Can you work these out from the model? Positions are in its coordinate system, mm. A direction names the side the tool comes from. Give positions to 0.01 mm unless a question says otherwise; leave off trailing zeros. Loops run counter-clockwise (first coordinate to the right, second up) from the corner with the lowest first, then second, coordinate; pieces in that order, holes last. Notation, with made-up numbers: (-3, 41) - (49, 41) arc R33 cw to (49, 77) - close; hole circle Ø7 at (67.5, 8.5). An arc over 180 degrees is marked (long way). Use a Markdown table: item, result. Add a question column.
```python
from build123d import *

# Parameters (mm, degrees)
SKETCH1_W           = 42
SKETCH1_H           = 42
BODY_DEPTH          = 48
CHAMFER1_SIZE       = 5.5
SKETCH2_R           = 2.5
SHAFT_DEPTH         = 22
SHAFTORIENTER_START = -15
SHAFTORIENTER_DEPTH = 15


with BuildPart() as part:
    # Sketch1 → Body (new body)
    with BuildSketch(Plane(origin=(0, 0, 0), x_dir=(1, 0, 0), z_dir=(0, 1, 0))):
        with Locations((21, 21)):
            Rectangle(SKETCH1_W, SKETCH1_H)
    extrude(amount=BODY_DEPTH)

    # Chamfer1
    chamfer1_edges = [part.edges().sort_by_distance(p)[0] for p in [
        (0, 24, -42),
        (42, 24, -42),
        (42, 24, 0),
        (0, 24, 0),
    ]]
    chamfer(chamfer1_edges, length=CHAMFER1_SIZE)

    # Sketch2 → Shaft (add)
    with BuildSketch(Plane(origin=(0, 48, 0), x_dir=(1, 0, 0), z_dir=(0, 1, 0))):
        with Locations(Location((21, 21, 0), (0, 0, 90))):
            Circle(SKETCH2_R)
    extrude(amount=SHAFT_DEPTH)

    # Sketch3 → ShaftOrienter (cut)
    with BuildSketch(Plane(origin=(0, 70, 0), x_dir=(1, 0, 0), z_dir=(0, 1, 0)).offset(SHAFTORIENTER_START)):
        with BuildLine():
            Line((23.05, 22.430908802), (23.05, 19.569091198))
            ThreePointArc((23.05, 19.569091198), (23.384848004, 20.25), (23.5, 21))
            ThreePointArc((23.5, 21), (23.384848004, 21.75), (23.05, 22.430908802))
        make_face()
    extrude(amount=SHAFTORIENTER_DEPTH, mode=Mode.SUBTRACT)


solid = part.part
```
1. Suppose I cut it at C-C (x = 21). List the corners of the cut face in (y, z) for me.
2. Suppose I cut it at B-B (z = -21). List the corners of the cut face in (x, y) for me.
3. Please list where these lines run through material, in increasing order: line 1 along Y through (x, z) = (19, -4.5); line 2 along X through (y, z) = (29, -5); line 3 along X through (y, z) = (66, -20). Write a range as [from, to].
4. Will these pins go through, and if not, where does the flat tip stop? P1, Ø3, axis at x = 23.5, z = -33, coming from the +Y side; P2, Ø10, axis at y = 57, z = -16, coming from the +X side; P3, Ø0.9, axis at y = 65.5, z = -21.5, coming from the +X side.
5. Suppose I cut it at A-A (y = 12). List the corners of the cut face in (x, z) for me.
6. Suppose I cut it at D-D (y = 56.5). List the corners of the cut face in (x, z) for me.
7. On a 3-axis mill with a long thin cutter (end or side, diameter ignored), from which of +Z, -Z, +X, -X, +Y, -Y can I reach the whole of each face in a straight line? I mean faces 1 (the face through (21, 70, -21)), 2 (the face through (23.05, 62, -21)), 3 (the face through (18.52, 58.85, -20.67)). Say none if no direction works.
Results below:
| question | item | result |
|---|---|---|
| 1 | outline | (0, -42) - (48, -42) - (48, -23.5) - (70, -23.5) - (70, -18.5) - (48, -18.5) - (48, 0) - (0, 0) - close |
| 2 | outline | (0, 0) - (42, 0) - (42, 48) - (23.5, 48) - (23.5, 55) - (23.05, 55) - (23.05, 70) - (18.5, 70) - (18.5, 48) - (0, 48) - close |
| 3 | line 1 | [0, 48] |
| 3 | line 2 | [0.5, 41.5] |
| 3 | line 3 | [18.71, 23.05] |
| 4 | P1 | y = 48 |
| 4 | P2 | x = 23.46 |
| 4 | P3 | x = 23.05 |
| 5 | outline | (0, -36.5) - (5.5, -42) - (36.5, -42) - (42, -36.5) - (42, -5.5) - (36.5, 0) - (5.5, 0) - (0, -5.5) - close |
| 6 | outline | (23.05, -22.43) - (23.05, -19.57) arc R2.5 ccw (long way) to start |
| 7 | face 1 | +Z, -Z, +X, -X, +Y |
| 7 | face 2 | +Z, -Z, +X, +Y |
| 7 | face 3 | +Y |
